Design review of the part built by this model. Coordinates are the model's own, in mm. A direction names the side the tool comes from. Coordinates: 2 decimals unless noted, no trailing zeros. Order: outer loops, then holes, each group sorted by start corner. A loop starts at its lowest first (then second) coordinate and runs counter-clockwise, first axis right, second up. Notation, with made-up numbers: M -26.5,-26.75 L 15.5,-26.75 A21 cw 15.5,9.25 Z; hole C 26,-6 d6. An arc over 180 degrees is marked long. Answer in a Markdown table with one row per item.
from build123d import *

# Parameters (mm, degrees)
SKETCH2_W             = 30
SKETCH2_H             = 200
BOSS_EXTRUDE1_DEPTH   = 10
SKETCH3_W             = 20
SKETCH3_H             = 30
SKETCH3_W_2           = 7
SKETCH3_H_2           = 104
CUT_EXTRUDE1_DEPTH    = 5
FILLET1_R             = 2.5
FILLET2_R             = 2.5
SKETCH4_W             = 3
SKETCH4_H             = 100
CUT_EXTRUDE2_DEPTH    = 10
FILLET3_R             = 1.5
F_3_0MM_DOWEL_HOLE1_D = 3


with BuildPart() as part:
    # Sketch2 → Boss-Extrude1 (new body)
    with BuildSketch(Plane(origin=(0, 0, 0), x_dir=(1, 0, 0), z_dir=(0, 1, 0))):
        Rectangle(SKETCH2_W, SKETCH2_H)
    extrude(amount=BOSS_EXTRUDE1_DEPTH)

    # Sketch3 → Cut-Extrude1 (cut)
    with BuildSketch(Plane(origin=(0, 10, 0), x_dir=(1, 0, 0), z_dir=(0, 1, 0))):
        with Locations((0, 85)):
            Rectangle(SKETCH3_W, SKETCH3_H)
        with Locations((0, -85)):
            Rectangle(SKETCH3_W, SKETCH3_H)
        with Locations((6.5, 0)):
            Rectangle(SKETCH3_W_2, SKETCH3_H_2)
        with Locations((-6.5, 0)):
            Rectangle(SKETCH3_W_2, SKETCH3_H_2)
    extrude(amount=-CUT_EXTRUDE1_DEPTH, mode=Mode.SUBTRACT)

    # Fillet1
    fillet1_edges = [part.edges().sort_by_distance(p)[0] for p in [
        (15, 5, 100),
        (-15, 5, 100),
        (-15, 5, -100),
        (15, 5, -100),
    ]]
    fillet(fillet1_edges, radius=FILLET1_R)

    # Fillet2
    fillet2_edges = [part.edges().sort_by_distance(p)[0] for p in [
        (0, 0, 100),
        (15, 0, 0),
        (-15, 0, 0),
        (0, 0, -100),
        (14.267766953, 0, -99.267766953),
        (-14.267766953, 0, -99.267766953),
        (14.267766953, 0, 99.267766953),
        (-14.267766953, 0, 99.267766953),
    ]]
    fillet(fillet2_edges, radius=FILLET2_R)

    # Sketch4 → Cut-Extrude2 (cut)
    with BuildSketch(Plane(origin=(0, 10, 0), x_dir=(1, 0, 0), z_dir=(0, 1, 0))):
        with Locations((6.5, 0)):
            Rectangle(SKETCH4_W, SKETCH4_H)
        with Locations((-6.5, 0)):
            Rectangle(SKETCH4_W, SKETCH4_H)
    extrude(amount=-CUT_EXTRUDE2_DEPTH, mode=Mode.SUBTRACT)

    # Fillet3
    fillet3_edges = [part.edges().sort_by_distance(p)[0] for p in [
        (5, 2.5, 50),
        (8, 2.5, 50),
        (5, 2.5, -50),
        (8, 2.5, -50),
        (-5, 2.5, 50),
        (-8, 2.5, 50),
        (-8, 2.5, -50),
        (-5, 2.5, -50),
    ]]
    fillet(fillet3_edges, radius=FILLET3_R - 0.0001)  # a hair under: the kernel refuses the full size

    # Ø3.0mm Dowel Hole1 (through all)
    with Locations(Plane(origin=(0, 5, 0), x_dir=(1, 0, 0), z_dir=(0, 1, 0))):
        with Locations((0, 92.5), (0, 77.5), (0, -77.5), (0, -92.5)):
            Hole(F_3_0MM_DOWEL_HOLE1_D / 2)


solid = part.part
(1) Insertion check: pin 1 Ø2.5 at (x, z) = (0, 92.5) entering from -Y; pin 2 Ø8 at (x, z) = (6.5, -18.5) entering from -Y; pin 3 Ø1.5 at (x, y) = (-3.5, 8) entering from -Z; pin 4 Ø6 at (x, z) = (2.5, 90) entering from +Y. Each pin has a flat end and moves straight along its axis. Give the tip position at first contact, or say it passes through.
Return value:
| item | result |
|---|---|
| pin 1 | passes through |
| pin 2 | stops at y = 0 |
| pin 3 | stops at z = -70 |
| pin 4 | stops at y = 5 |
(2) Draft analysis for pull direction Z (two halves, no side actions). For faces 1 (the flat face through (-0.2, 4.5, -100)), 2 (the flat face through (10, 8, 85)), 3 (the flat face through (10, 8, 1)), state which applies: pulls with the +Z half, pulls with the -Z half, needs draft (parallel to the pull), parting line crosses it, or undercut.
Return value:
| item | result |
|---|---|
| face 1 | pulls with the -Z half |
| face 2 | needs draft |
| face 3 | undercut |
(3) Add section A-A, the plane z = -24.5. Give the boundary of the cut face in (x, y).
Return value:
| item | result |
|---|---|
| outline | M -15,2.5 A2.5 ccw -12.5,0 L -8,0 L -8,5 L -10,5 L -10,10 L -15,10 Z; M -5,0 L 5,0 L 5,5 L 3,5 L 3,10 L -3,10 L -3,5 L -5,5 Z; M 8,0 L 12.5,0 A2.5 ccw 15,2.5 L 15,10 L 10,10 L 10,5 L 8,5 Z |
(4) For line 1 along Z through (x, y) = (0, 3.2); line 2 along X through (y, z) = (5.5, 28); line 3 along X through (y, z) = (3.1, -77.5), list the stretches that pass through material, from the lowest coordinate up. Write a range as from..to.
Return value:
| item | result |
|---|---|
| line 1 | z = -100..-94, -91..-79, -76..76, 79..91, 94..100 |
| line 2 | x = -15..-10, -3..3, 10..15 |
| line 3 | x = -15..-1.5, 1.5..15 |
(5) For faces 4 (the flat face through (-7, 8, -52)), 5 (the flat face through (-8, 3, 1)), 6 (the flat face through (-10, 8, 85)), 7 (the flat face through (0, 8, -70)), list the 3-axis set-ups (+Z, -Z, +X, -X, +Y, -Y) from which the entire face can be reached by the end or side of a thin tool; tool diameter is ignored.
Return value:
| item | result |
|---|---|
| face 4 | +Y |
| face 5 | +Y, -Y |
| face 6 | +Z, +Y |
| face 7 | -Z, +Y |
(6) Add section B-B, the plane y = 6.5. Give the boundary of the cut face in (x, z).
Return value:
| item | result |
|---|---|
| outline | M -15,-97.5 A2.5 ccw -12.5,-100 L -10,-100 L -10,-70 L 10,-70 L 10,-100 L 12.5,-100 A2.5 ccw 15,-97.5 L 15,97.5 A2.5 ccw 12.5,100 L 10,100 L 10,70 L -10,70 L -10,100 L -12.5,100 A2.5 ccw -15,97.5 Z; hole M -10,-52 L -3,-52 L -3,52 L -10,52 Z; hole M 3,-52 L 10,-52 L 10,52 L 3,52 Z |
